Could you check a few things on this model? Use its own coordinates, in mm. A direction names the side the tool comes from. Coordinates: 2 decimals unless noted, no trailing zeros. Loops run counter-clockwise (first coordinate to the right, second up) from the corner with the lowest first, then second, coordinate; pieces in that order, holes last. Notation, with made-up numbers: (73, 70) - (97, 70) arc R17 ccw to (97, 85) - close; hole circle Ø4 at (39.25, 44). An arc over 180 degrees is marked (long way). Use CSV: the item, a comma, the result in double quotes.
from build123d import *

# Parameters (mm, degrees)
BOSS_EXTRUDE1_DEPTH = 57.15
BOSS_EXTRUDE2_DEPTH = 12.7
CUT_EXTRUDE1_DEPTH  = 25.4


with BuildPart() as part:
    # Sketch1 → Boss-Extrude1 (new body, symmetric)
    with BuildSketch(Plane(origin=(0, 0, 0), x_dir=(0, 0, -1), z_dir=(1, 0, 0))):
        Polygon((-28.575, 0), (28.575, 0), (28.575, 31.75), (-12.7, 31.75), (-12.7, 12.7), (-28.575, 12.7), align=None)
    extrude(amount=BOSS_EXTRUDE1_DEPTH, both=True)

    # Sketch2 → Boss-Extrude2 (add)
    with BuildSketch(Plane(origin=(0, 31.75, 0), x_dir=(1, 0, 0), z_dir=(0, 1, 0))):
        Polygon((-28.575, 28.575), (28.575, 28.575), (28.575, 9.525), (19.05, 9.525), (19.05, 19.05), (-19.05, 19.05), (-19.05, 9.525), (-28.575, 9.525), align=None)
    extrude(amount=BOSS_EXTRUDE2_DEPTH)

    # Sketch3 → Cut-Extrude1 (cut)
    with BuildSketch(Plane(origin=(0, 44.45, 0), x_dir=(1, 0, 0), z_dir=(0, 1, 0))):
        Polygon((-38.1, 9.525), (-19.05, 9.525), (-19.05, 19.05), (19.05, 19.05), (19.05, 9.525), (38.1, 9.525), (38.1, -12.7), (-38.1, -12.7), align=None)
    extrude(amount=-CUT_EXTRUDE1_DEPTH, mode=Mode.SUBTRACT)


solid = part.part
(1) Suppose I cut it at A-A (x = 4.5). Write out the boundary of the cut face in (y, z) (3 decimals), plus the area to 3 significant figures.
Computed:
outline,"(0, -28.575) - (44.45, -28.575) - (44.45, -19.05) - (19.05, -19.05) - (19.05, 12.7) - (12.7, 12.7) - (12.7, 28.575) - (0, 28.575) - close"
area,"1,230 mm²"
(2) Please list where these lines run through material, in increasing order: line 1 (X direction, y = 22, z = -2.5); line 2 (Y direction, x = -44, z = 4); line 3 (Z direction, x = 51, y = 28) (3 decimals).
Computed:
line 1,"x = -57.15 to -38.1, 38.1 to 57.15"
line 2,"y = 0 to 31.75"
line 3,"z = -28.575 to 12.7"
(3) Which directions (+Z, -Z, +X, -X, +Y, -Y) give clear straight access to the entire face, cutting with the end or side of a thin tool? Please do faces 4 (the face through (1, 0, 0)), 5 (the face through (1, 12.7, 21)), 6 (the face through (-57.15, 16, -6)), 7 (the face through (46, 31.75, -8)), 8 (the face through (0, 32, -19.05)).
Computed:
face 4,"+Z, -Z, +X, -X, -Y"
face 5,"+Z, +X, -X, +Y"
face 6,"+Z, -Z, -X, +Y, -Y"
face 7,"+Z, -Z, +X, +Y"
face 8,"+Z, +Y"
(4) Suppose I cut it at D-D (y = 27). Write out the boundary of the cut face in (x, z) (3 decimals), plus the area to 3 significant figures.
Computed:
outline,"(-57.15, -28.575) - (57.15, -28.575) - (57.15, 12.7) - (38.1, 12.7) - (38.1, -9.525) - (19.05, -9.525) - (19.05, -19.05) - (-19.05, -19.05) - (-19.05, -9.525) - (-38.1, -9.525) - (-38.1, 12.7) - (-57.15, 12.7) - close"
area,"2,660 mm²"
(5) Thinking about a two-plate mould opening in X: for faces 1 (the face through (-28.575, 38, -19)), 2 (the face through (1, 6, 28.575)), 3 (the face through (-27, 29, -9.525)), which applies, +X half, -X half, draft (parallel to the pull), parting line (faces both ways), or undercut?
Computed:
face 1,"-X half"
face 2,"draft"
face 3,"undercut"
(6) Suppose I cut it at C-C (z = -12). Write out the boundary of the cut face in (x, y) (3 decimals).
Computed:
outline,"(-57.15, 0) - (57.15, 0) - (57.15, 31.75) - (28.575, 31.75) - (28.575, 44.45) - (19.05, 44.45) - (19.05, 19.05) - (-19.05, 19.05) - (-19.05, 44.45) - (-28.575, 44.45) - (-28.575, 31.75) - (-57.15, 31.75) - close"
(7) Will these pins go through, and if not, where does the flat tip stop? pin 1 (9.5 mm diameter, centred on x = -26.5, y = 36.5, fed in from +Z) (3 decimals); pin 2 (6.5 mm diameter, centred on y = 40, z = -17.5, fed in from +X) (3 decimals); pin 3 (5 mm diameter, centred on x = 29.5, y = 17.5, fed in from +Z).
Computed:
pin 1,"stops at z = -9.525"
pin 2,"stops at x = 28.575"
pin 3,"stops at z = 12.7"
(8) Suppose I cut it at B-B (y = 35.5). Write out the boundary of the cut face in (x, z) (3 decimals), plus the area to 3 significant figures.
Computed:
outline,"(-28.575, -28.575) - (28.575, -28.575) - (28.575, -9.525) - (19.05, -9.525) - (19.05, -19.05) - (-19.05, -19.05) - (-19.05, -9.525) - (-28.575, -9.525) - close"
area,"726 mm²"
